Here's how the part is built. I have some questions about the finished solid (model axes, mm). Round coordinates to 2 decimals unless told otherwise and drop trailing zeros. Order: outer loops, then holes, each group sorted by start corner. A loop starts at its lowest first (then second) coordinate and runs counter-clockwise, first axis right, second up. Notation, with made-up numbers: (12.5, 47) - (44.5, 47) arc R25 cw to (44.5, 64) - close; hole circle Ø9 at (9.25, -1.5). An arc over 180 degrees is marked (long way). Answer as a JSON object with one key per item and string values.
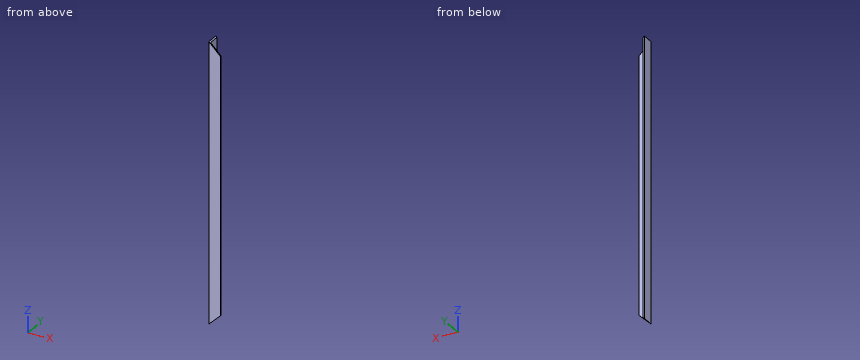
Autodesk Inventor part; units mm, degrees
ref_plane "YZ Plane" through (0, 0, 0) normal (1, 0, 0) x (0, 1, 0)
ref_plane "XZ Plane" through (0, 0, 0) normal (0, 1, 0) x (-1, 0, 0)
ref_plane "XY Plane" through (0, 0, 0) normal (0, 0, 1) x (1, 0, 0)
sketch "Sketch1" plane through (0, 0, 0) normal (0, 0, 1) x (1, 0, 0)
  line L0 (0, 0) -> (0, 50.8)
  line L1 (0, 50.8) -> (4.7625, 50.8)
  line L2 (4.7625, 50.8) -> (4.7625, 4.7625)
  line L3 (4.7625, 4.7625) -> (50.8, 4.7625)
  line L4 (50.8, 4.7625) -> (50.8, 0)
  line L5 (50.8, 0) -> (0, 0)
  dimension "d0" = 4.7625
  dimension "d1" = 50.8
  dimension "d2" = 4.7625
  dimension "d3" = 50.8
extrude "Extrusion1" add sketch "Sketch1" along normal blind 1244.6
sketch "Sketch5" plane through (0, 0, 0) normal (0, -1, 0) x (1, 0, 0)
  line L0 (50.8, 1244.6) -> (0, 1244.6)
  line L1 (50.8, 0) -> (0, 0)
  line L2 (50.8, 0) -> (50.8, 1244.6)
  line L3 (0, 1244.6) -> (50.8, 1193.8)
  line L4 (0, 0) -> (50.8, 50.8)
  dimension "d16" = 45
  dimension "d17" = 45
extrude "Extrusion5" cut sketch "Sketch5" against normal blind 50.8 contours L2 L3 L0
sketch "Sketch6" plane through (0, 0, 0) normal (0, -1, 0) x (1, 0, 0)
  line L0 (0, 0) -> (0, 1244.6)
  line L1 (50.8, 0) -> (0, 0)
  line L2 (50.8, 0) -> (50.8, 1193.8)
  line L3 (0, 0) -> (50.8, 50.8)
  dimension "d20" = 45
extrude "Extrusion6" cut sketch "Sketch6" against normal blind 50.8
properties part number "BOXC_L49"
1. Imagine slicing it at C-C (y = 22). List the corners of the cut face in (x, z) for me, plus the area to 3 significant figures.
Responses:
{"outline": "(0, 0) - (4.76, 4.76) - (4.76, 1239.84) - (0, 1244.6) - close", "area": "5,900 mm2"}
2. Imagine slicing it at A-A (z = 146). List the corners of the cut face in (x, y) for me.
Responses:
{"outline": "(0, 0) - (50.8, 0) - (50.8, 4.76) - (4.76, 4.76) - (4.76, 50.8) - (0, 50.8) - close"}
3. If I drill on L1, parallel to X at y = 42.5, z = 479.5, over which ranges is the centre line in solid material (lowest first)? Write a range as [from, to].
Responses:
{"L1": "[0, 4.76]"}
4. For P1, Ø8, axis at y = 11.5, z = 720, coming from the +X side; P2, Ø1, axis at x = 42, z = 366.5, coming from the +Y side, each with a flat end and sliding along its axis, tell me the tip position at first contact or that it passes through.
Responses:
{"P1": "x = 4.76", "P2": "y = 4.76"}
5. Imagine slicing it at B-B (x = 34). List the corners of the cut face in (y, z) for me, plus the area to 3 significant figures.
Responses:
{"outline": "(0, 34) - (4.76, 34) - (4.76, 1210.6) - (0, 1210.6) - close", "area": "5,600 mm2"}
